Could you check a few things on this model? Use its own coordinates, in mm. A direction names the side the tool comes from. Give positions to 0.01 mm unless a question says otherwise; leave off trailing zeros. Write each loop counter-clockwise with the first axis right and the second up, starting at its lowest first coordinate (ties: lowest second). Pieces come first, ordered by that corner, then holes. Notation, with made-up numbers: (77, 46) - (81, 46) arc R29 cw to (81, 82) - close; hole circle Ø11 at (4.5, 27). An arc over 180 degrees is marked (long way). Write item = value, one per line.
from build123d import *

# Parameters (mm, degrees)
F0_W     = 20.6375
F0_H     = 6.35
F1_DEPTH = 11.27125
F2_R     = 1.7272
F3_DEPTH = 6.35
F4_R     = 1.35255
F5_DEPTH = 4.7625
F6_SIZE  = 4.7625


with BuildPart() as f1:
    # F0 (on Top) → F1 (new body)
    with BuildSketch(Plane.XY):
        with Locations((10.31875, 3.175)):
            Rectangle(F0_W, F0_H)
    extrude(amount=F1_DEPTH)

    # F2 (on face) → F3 (cut, through all)
    with BuildSketch(Plane.XZ):
        with Locations((10.31875, 7.3025)):
            Circle(F2_R)
    extrude(amount=-F3_DEPTH, mode=Mode.SUBTRACT)

    # F4 (on face) → F5 (cut)
    with BuildSketch(Plane(origin=(0, 0, 0), x_dir=(1, 0, 0), z_dir=(0, 0, -1))):
        with Locations((3.175, -3.175)):
            Circle(F4_R)
        with Locations((17.4625, -3.175)):
            Circle(F4_R)
    extrude(amount=-F5_DEPTH, mode=Mode.SUBTRACT)

    # F6
    f6_edges = [f1.edges().sort_by_distance(p)[0] for p in [
        (0, 3.175, 11.27125),
        (20.6375, 3.175, 11.27125),
    ]]
    chamfer(f6_edges, length=F6_SIZE)


solid = f1.part
1. If we section it at D-D, the plane z = 2.5: Count the separate pieces of the cut face and the enclosed holes in it, and give its area (3 significant figures).
Filled sheet:
separate_pieces = 1
enclosed_holes = 2
area = 120 mm2
2. Which directions (+Z, -Z, +X, -X, +Y, -Y) give clear straight access to the entire face, cutting with the end or side of a thin tool? Please do faces 1 (the face through (10, 6.35, 4)), 2 (the face through (3, 3, 4.762)).
Filled sheet:
face_1 = +Z, -Z, +X, -X, +Y
face_2 = -Z
3. If we section it at A-A, the plane z = 8: Please give me the cut outline in (x, y).
Filled sheet:
outline = (1.49, 0) - (8.74, 0) - (8.74, 6.35) - (1.49, 6.35) - close; (11.9, 0) - (19.15, 0) - (19.15, 6.35) - (11.9, 6.35) - close
4. Thinking about a two-plate mould opening in Z: for faces 3 (the face through (18.29, 3.131, 8.857)), 4 (the face through (17, 3, 4.762)), 5 (the face through (2.102, 3.998, 2.348)), 6 (the face through (11.116, 3.131, 5.77)), which applies, pulls with the +Z half, pulls with the -Z half, needs draft (parallel to the pull), parting line crosses it, or undercut?
Filled sheet:
face_3 = pulls with the +Z half
face_4 = pulls with the -Z half
face_5 = needs draft
face_6 = undercut
5. I need wall thicknesses on line 1 (Z direction, x = 10.75, y = 3.5) (3 decimals); line 2 (Y direction, x = 2.5, z = 2.5); line 3 (Z direction, x = 9.5, y = 1.75). Which ranges of each line are inside material? Lowest first, please.
Filled sheet:
line_1 = 0 to 5.63, 8.975 to 11.271
line_2 = 0 to 2, 4.35 to 6.35
line_3 = 0 to 5.78, 8.82 to 11.27
6. If we section it at C-C, the plane x = 9: Please give me the cut outline in (y, z).
Filled sheet:
outline = (0, 0) - (6.35, 0) - (6.35, 6.19) - (0, 6.19) - close; (0, 8.42) - (6.35, 8.42) - (6.35, 11.27) - (0, 11.27) - close
7. For pin 1 (1.4 mm diameter, centred on x = 17.5, y = 3.5, fed in from -Z); pin 2 (2.5 mm diameter, centred on x = 3.175, y = 3.175, fed in from +Z); pin 3 (3 mm diameter, centred on x = 10.32, z = 7.3, fed in from +Y), each with a flat end and sliding along its axis, tell me the tip position at first contact or that it passes through.
Filled sheet:
pin_1 = 4.76
pin_2 = 10.93
pin_3 = through
8. If we section it at B-B, the plane y = 2.25: Please give me the cut outline in (x, z) (1 decimal).
Filled sheet:
outline = (0, 0) - (2.2, 0) - (2.2, 4.8) - (4.2, 4.8) - (4.2, 0) - (16.5, 0) - (16.5, 4.8) - (18.4, 4.8) - (18.4, 0) - (20.6, 0) - (20.6, 6.5) - (15.9, 11.3) - (4.8, 11.3) - (0, 6.5) - close; hole circle Ø3.5 at (10.3, 7.3)
